Autodesk Inventor part; units mm, degrees
ref_plane "YZ Plane" through (0, 0, 0) normal (1, 0, 0) x (0, 1, 0)
ref_plane "XZ Plane" through (0, 0, 0) normal (0, 1, 0) x (-1, 0, 0)
ref_plane "XY Plane" through (0, 0, 0) normal (0, 0, 1) x (1, 0, 0)
sketch "Sketch1" plane through (0, 0, 0) normal (1, 0, 0) x (0, 1, 0)
  line L0 (7.9725, -6.9898) -> (-601.6275, -6.9898)
  line L1 (-601.6275, -6.9898) -> (-601.6275, -159.3898)
  line L2 (-601.6275, -159.3898) -> (7.9725, -159.3898)
  line L3 (7.9725, -159.3898) -> (7.9725, -6.9898)
  point P0 (0, 0)
  dimension "d0" = 609.6
  dimension "d1" = 152.4
extrude "Extrusion1" add sketch "Sketch1" along normal blind 88.9
sketch "Sketch2" plane through (0, -601.6275, -6.9898) normal (0, 0, 1) x (1, 0, 0)
  line L0 (0, 0) -> (0, 609.6)
  line L1 (0, 609.6) -> (0, 393.7)
  line L2 (0, 0) -> (88.9, 0)
  line L3 (0, 0) -> (0, 215.9)
  line L4 (88.9, 0) -> (88.9, 609.6)
  line L5 (0, 393.7) -> (88.9, 393.7)
  line L6 (88.9, 393.7) -> (88.9, 215.9)
  line L7 (88.9, 215.9) -> (0, 215.9)
  line L8 (0, 215.9) -> (0, 393.7)
  line L9 (0, 393.7) -> (0, 215.9)
  point P0 (0, 601.6275)
  point P1 (0, 215.9)
  dimension "d4" = 215.9
  dimension "d5" = 215.9
extrude "Extrusion2" cut sketch "Sketch2" against normal blind 76.2 contours L0 L5 L4 L7
sketch "Sketch3" plane through (88.9, 0, 0) normal (1, 0, 0) x (0, 0, -1)
  point P0 (0, 0)
sketch "Sketch4" plane through (0, -601.6275, -6.9898) normal (0, 0, 1) x (1, 0, 0)
  line L0 (18.9312, 116.4608) -> (72.6429, 116.4608)
  line L1 (72.6429, 116.4608) -> (72.6429, 86.5231)
  line L2 (72.6429, 86.5231) -> (18.9312, 86.5231)
  line L3 (18.9312, 86.5231) -> (18.9312, 116.4608)
  point P0 (0, 601.6275)
extrude "Extrusion3" add sketch "Sketch4" along normal blind 101.6
sketch "Sketch5" plane through (72.6429, -515.1044, -6.9898) normal (1, 0, 0) x (0, 0, -1)
  line L0 (-101.6, 0) -> (-66.3848, 29.9377)
  line L1 (0, 29.9377) -> (-101.6, 29.9377)
  line L2 (-101.6, 0) -> (-101.6, 29.9377)
  line L3 (-101.6, 0) -> (-101.6, 29.9377)
  point P0 (-6.9898, 515.1044)
extrude "Extrusion4" cut sketch "Sketch5" against normal through all
sketch "Sketch6" plane through (18.9312, -515.1044, 94.6102) normal (0, 0.7618887, 0.647708) x (1, 0, 0)
  line L0 (0, 46.221) -> (53.7117, 46.221)
  line L1 (53.7117, 77.4079) -> (53.7117, 0)
  line L2 (0, 46.221) -> (53.7117, 46.221)
  line L3 (53.7117, 46.221) -> (53.7117, 0)
  line L4 (53.7117, 0) -> (0, 0)
  line L5 (0, 0) -> (0, 46.221)
  point P0 (-18.9312, 405.7197)
extrude "Extrusion5" add sketch "Sketch6" along normal blind 165.1
sketch "Sketch7" plane through (72.6429, -515.1044, -6.9898) normal (1, 0, 0) x (0, 0, -1)
  point P0 (-6.9898, 515.1044)
sketch "Sketch8" plane through (72.6429, -515.1044, -6.9898) normal (1, 0, 0) x (0, 0, -1)
  line L0 (-173.3214, 155.7255) -> (-208.5366, 125.7878)
  line L1 (-208.5366, 125.7878) -> (-147.8703, 125.7878)
  line L2 (-66.3848, 29.9377) -> (-173.3214, 155.7255)
  line L3 (-173.3214, 155.7255) -> (-208.5366, 125.7878)
  line L4 (-147.8703, 125.7878) -> (-173.3214, 155.7255)
  point P0 (-6.9898, 515.1044)
extrude "Extrusion6" cut sketch "Sketch8" against normal through all
sketch "Sketch9" plane through (72.6429, -389.3166, 201.5467) normal (0, 1, 0) x (1, 0, 0)
  point P0 (-72.6429, 201.5467)
sketch "Sketch10" plane through (0, -385.7275, -6.9898) normal (0, 1, 0) x (1, 0, 0)
  point P0 (0, -6.9898)
sketch "Sketch11" plane through (0, -385.7275, -6.9898) normal (0, 1, 0) x (1, 0, 0)
  point P0 (0, -6.9898)
sketch "Sketch12" plane through (0, -385.7275, -6.9898) normal (0, 1, 0) x (1, 0, 0)
  point P0 (0, -6.9898)
sketch "Sketch13" plane through (0, 0, 0) normal (-1, 0, 0) x (0, 0, 1)
  point P0 (0, 0)
sketch "Sketch14" plane through (0, -385.7275, -6.9898) normal (0, 1, 0) x (1, 0, 0)
  line L0 (88.9, 76.2) -> (0, 76.2)
  line L1 (0, 0) -> (0, 76.2)
  line L2 (88.9, 76.2) -> (0, 76.2)
  line L3 (88.9, 76.2) -> (88.9, 0)
  line L4 (0, 76.2) -> (88.9, 76.2)
  line L5 (88.9, 76.2) -> (0, 76.2)
  line L6 (0, 76.2) -> (0, 0)
  line L7 (0, 0) -> (88.9, 0)
  line L8 (88.9, 0) -> (88.9, 76.2)
  point P0 (0, -6.9898)
sketch "Sketch15" plane through (0, -385.7275, -6.9898) normal (0, 1, 0) x (1, 0, 0)
  line L0 (88.9, 76.2) -> (88.9, 0)
  line L1 (88.9, 38.1) -> (0, 38.1)
  line L2 (0, 0) -> (0, 76.2)
  line L3 (88.9, 76.2) -> (0, 76.2)
  circle A0 centre (63.5, 38.1) radius 6.35
  circle A1 centre (25.4, 38.1) radius 6.35
  point P0 (0, -6.9898)
  dimension "d20" = 12.7
  dimension "d21" = 12.7
extrude "Extrusion7" add sketch "Sketch15" along normal blind 177.8 contours A0 L1 | L1 A0 | A1 L1 | L1 A1
sketch "Sketch16" plane through (0, 7.9725, -6.9898) normal (0, 1, 0) x (1, 0, 0)
  line L0 (29.6959, 92.8158) -> (65.2559, 92.8158)
  line L1 (65.2559, 92.8158) -> (65.2559, 57.2558)
  line L2 (65.2559, 57.2558) -> (29.6959, 57.2558)
  line L3 (29.6959, 57.2558) -> (29.6959, 92.8158)
  point P0 (0, -6.9898)
  dimension "d24" = 35.56
  dimension "d25" = 35.56
extrude "Extrusion8" add sketch "Sketch16" along normal blind 127
sketch "Sketch17" plane through (29.6959, 7.9725, -64.2457) normal (0, 0, 1) x (1, 0, 0)
  line L0 (0, 127) -> (35.56, 127)
  line L1 (35.56, 0) -> (35.56, 127)
  line L2 (0, 127) -> (35.56, 127)
  line L3 (35.56, 127) -> (35.56, 91.44)
  line L4 (35.56, 91.44) -> (0, 91.44)
  line L5 (0, 91.44) -> (0, 127)
  point P0 (-29.6959, -7.9725)
  dimension "d28" = 35.56
extrude "Extrusion9" add sketch "Sketch17" along normal blind 127
sketch "Sketch18" plane through (65.2559, 7.9725, -64.2457) normal (1, 0, 0) x (0, 0, -1)
  line L0 (0, 91.44) -> (-127, 91.44)
  line L1 (-64.2457, 91.44) -> (-45.72, 127)
  line L2 (35.56, 127) -> (-127, 127)
  line L3 (-45.72, 127) -> (-127, 127)
  line L4 (-127, 127) -> (-127, 91.44)
  line L5 (-127, 91.44) -> (-64.2457, 91.44)
  line L6 (-127, 127) -> (-127, 91.44)
  line L7 (35.56, 127) -> (-127, 127)
  line L8 (0, 127) -> (-14.8626, 91.44)
  line L9 (-64.2457, 91.44) -> (-14.8626, 91.44)
  line L10 (-14.8626, 91.44) -> (0, 127)
  line L11 (-45.72, 127) -> (-127, 127)
  line L12 (0, 127) -> (-49.9714, 127)
  point P0 (-64.2457, -7.9725)
extrude "Extrusion10" cut sketch "Sketch18" against normal through all contours L0 L4 L2 L1
sketch "Sketch19" plane through (65.2559, 7.9725, -64.2457) normal (1, 0, 0) x (0, 0, -1)
  line L0 (0, 91.44) -> (-64.2457, 91.44)
  line L1 (-32.1228, 91.44) -> (-14.9944, 127)
  line L2 (35.56, 127) -> (-45.72, 127)
  line L3 (-32.1228, 91.44) -> (-64.2457, 91.44)
  line L4 (-64.2457, 91.44) -> (-45.72, 127)
  line L5 (-64.2457, 91.44) -> (-45.72, 127)
  line L6 (-45.72, 127) -> (-14.9944, 127)
  point P0 (-64.2457, -7.9725)
extrude "Extrusion11" cut sketch "Sketch19" against normal through all
sketch "Sketch20" plane through (65.2559, 7.9725, -64.2457) normal (1, 0, 0) x (0, 0, -1)
  line L0 (35.56, 127) -> (-14.9944, 127)
  line L1 (-0.2658, 127) -> (-21.0098, 91.44)
  line L2 (0, 91.44) -> (-32.1228, 91.44)
  line L3 (-21.0098, 91.44) -> (-32.1228, 91.44)
  line L4 (-32.1228, 91.44) -> (-14.9944, 127)
  line L5 (-32.1228, 91.44) -> (-14.9944, 127)
  line L6 (-14.9944, 127) -> (-0.2658, 127)
  point P0 (-64.2457, -7.9725)
extrude "Extrusion12" cut sketch "Sketch20" against normal through all
sketch "Sketch21" plane through (0, 7.9725, -6.9898) normal (0, 1, 0) x (1, 0, 0)
  point P0 (0, -6.9898)
sketch "Sketch22" plane through (65.2559, 7.9725, -64.2457) normal (1, 0, 0) x (0, 0, -1)
  line L0 (-0.2658, 127) -> (-21.0098, 91.44)
  line L1 (-21.0098, 91.44) -> (-0.2658, 127)
  line L2 (-0.2658, 127) -> (16.5705, 127)
  line L3 (35.56, 127) -> (-0.2658, 127)
  line L4 (0, 0) -> (0, 91.44)
  line L5 (0, 91.44) -> (16.5705, 127)
  line L6 (0, 91.44) -> (-21.0098, 91.44)
  line L7 (0, 91.44) -> (-21.0098, 91.44)
  point P0 (-64.2457, -7.9725)
extrude "Extrusion13" cut sketch "Sketch22" against normal through all
sketch "Sketch23" plane through (0, -385.7275, -6.9898) normal (0, 1, 0) x (1, 0, 0)
  point P0 (0, -6.9898)
sketch "Sketch24" plane through (0, -601.6275, -159.3898) normal (0, -1, 0) x (1, 0, 0)
  line L0 (0, 152.4) -> (88.9, 152.4)
  line L1 (88.9, 152.4) -> (88.9, 0)
  line L2 (0, 0) -> (88.9, 0)
  line L3 (0, 76.2) -> (88.9, 76.2)
  circle A0 centre (44.45, 76.2) radius 25.4
  point P0 (0, 159.3898)
extrude "Extrusion14" add sketch "Sketch24" along normal blind 12.7
properties part number "exploration cuboid" material "Silicon Nitride"
Input: part model. Units: mm. Frame: model coordinates. A direction names the side the tool comes from. Give positions to 0.01 mm unless a question says otherwise; leave off trailing zeros. Loops run counter-clockwise (first coordinate to the right, second up) from the corner with the lowest first, then second, coordinate; pieces in that order, holes last.
1) Section query B-B on z = 29.5. Return the cut outline in (x, y).
A:
outline: (18.93, -515.1) - (72.64, -515.1) - (72.64, -485.17) - (18.93, -485.17) - close
2) Reachability of faces 4 (the flat face through (29.696, 71, -82)), 5 (the flat face through (72.643, -461, 105)), 6 (the cylindrical face through (38.944, -607.889, -58.394)) from +Z, -Z, +X, -X, +Y, -Y: full face, straight path, thin tool, end or side. Return the list, or none.
A:
face 4: +Z, -Z, -X, +Y
face 5: +Z, +X, +Y, -Y
face 6: -Y
3) Section query C-C on y = -101. Return the cut outline in (x, z).
A:
outline: (0, -159.39) - (88.9, -159.39) - (88.9, -6.99) - (0, -6.99) - close
4) Line query: L1, parallel to Y at x = 67, z = -25.5; L2, parallel to Z at x = 45.5, y = -281; L3, parallel to Y at x = 43, z = -3.5. Output: solid intervals per line, ascending.
A:
L1: y = -601.63 to -385.73, -207.93 to 7.97
L2: z = -159.39 to -83.19
L3: y = -515.1 to -485.17
5) Contact query for flat-ended pins moving along their axis: pin 1 (1.5 mm diameter, centred on y = -460, z = -59, fed in from -X); pin 2 (2 mm diameter, centred on x = 11.5, z = -23, fed in from +Y); pin 3 (3 mm diameter, centred on x = 64, y = -386.5, fed in from +Z); pin 4 (12 mm diameter, centred on x = 28.5, z = -26, fed in from -Y). Output: stop coordinate, or through.
A:
pin 1: stops at x = 0
pin 2: stops at y = 7.97
pin 3: stops at z = -6.99
pin 4: stops at y = -601.63
6) Section query A-A on x = 81. Return the cut outline in (y, z).
A:
outline: (-601.63, -159.39) - (7.97, -159.39) - (7.97, -6.99) - (-207.93, -6.99) - (-207.93, -83.19) - (-385.73, -83.19) - (-385.73, -6.99) - (-601.63, -6.99) - close
7) Mould query, pull axis Z, two halves, no side actions, for faces 1 (the flat face through (45.41, -437.91, 99.57)), 2 (the flat face through (47, 71, -99.806)), 3 (the flat face through (65.256, 71, -82)). Classes: released by +Z, released by -Z, zero draft, split by the parting line, or undercut.
A:
face 1: undercut
face 2: released by -Z
face 3: zero draft
8) Section query D-D on x = 44.45. Return the cut outline in (y, z) (1 decimal), and give its area (3 significant figures).
A:
outline: (-614.3, -108.6) - (-601.6, -108.6) - (-601.6, -159.4) - (8, -159.4) - (8, -99.8) - (135, -99.8) - (135, -80.8) - (99.4, -64.2) - (8, -64.2) - (8, -7) - (-207.9, -7) - (-207.9, -83.2) - (-385.7, -83.2) - (-385.7, -7) - (-485.2, -7) - (-485.2, 59.4) - (-389.3, 140.9) - (-389.3, 201.5) - (-515.1, 94.6) - (-515.1, -7) - (-601.6, -7) - (-601.6, -57.8) - (-614.3, -57.8) - close
area: 93,500 mm2
